Here's how the part is built. I have some questions about the finished solid (model axes, mm). Face numbers are marked on the shaded views. A direction names the side the tool comes from. Give positions to 0.01 mm unless a question says otherwise; leave off trailing zeros. Write each loop counter-clockwise with the first axis right and the second up, starting at its lowest first coordinate (ties: lowest second). Pieces come first, ordered by that corner, then holes. Notation, with made-up numbers: (52, 24) - (57, 24) arc R19 ccw to (57, 49) - close; hole circle Ø6 at (82, 69.5). An arc over 180 degrees is marked (long way). Use one line per item in the form item = value. Start each with the question number.
from build123d import *

# Parameters (mm, degrees)
BOSS_EXTRUDE1_DEPTH      = 4
BOSS_EXTRUDE1_DEPTH_BACK = 2


with BuildPart() as part:
    # Sketch3 → Boss-Extrude1 (new body, two sides)
    with BuildSketch(Plane.XY) as boss_extrude1_sk:
        with BuildLine():
            Line((-3.803846336, 5.696775672), (24.708284265, 24.734871916))
            ThreePointArc((24.708284265, 24.734871916), (65.032506622, 5.199104), (28.324251817, -20.49512037))
            Line((28.324251817, -20.49512037), (-2.850444576, -6.228761171))
            ThreePointArc((-2.850444576, -6.228761171), (-6.828213831, -0.545889982), (-3.803846336, 5.696775672))
        make_face()
        with BuildLine():
            Line((-3.526193319, 5.28095263), (24.985937282, 24.319048874))
            ThreePointArc((24.985937282, 24.319048874), (64.534096854, 5.159258016), (28.532313465, -20.04046627))
            Line((28.532313465, -20.04046627), (-2.642382928, -5.774107071))
            ThreePointArc((-2.642382928, -5.774107071), (-6.329804063, -0.506043998), (-3.526193319, 5.28095263))
        make_face(mode=Mode.SUBTRACT)
    extrude(amount=BOSS_EXTRUDE1_DEPTH)
    extrude(boss_extrude1_sk.sketch, amount=-BOSS_EXTRUDE1_DEPTH_BACK)


solid = part.part
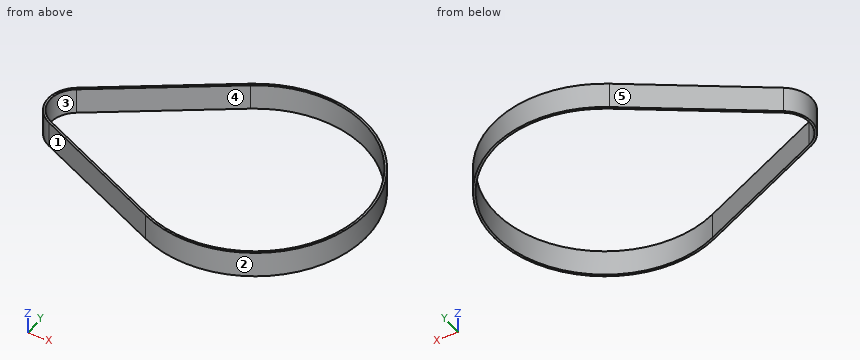
1. I want a section at C-C, the plane y = -3.5. List the corners of the cut face in (x, z) for me.
2. I want a section at A-A, the plane x = 59.5. List the corners of the cut face in (y, z) for me.
3. I want a section at B-B, the plane z = 2.9. List the corners of the cut face in (x, y) for me, then the cut area to 3 significant figures.
4. For P1, Ø1.5, axis at y = 21, z = 2.5, coming from the -X side; P2, Ø3, axis at y = -14.5, z = 0.5, coming from the +X side; P3, Ø1.5, axis at y = 7, z = 0.5, coming from the +X side, each with a flat end and sliding along its axis, tell me the tip position at first contact or that it passes through.
5. We'd pull the mould along X, two halves only. Please class the marked faces 1, 2 and 3: pulls with the +X half, pulls with the -X half, needs draft (parallel to the pull), parting line crosses it, or undercut.
6. For the marked faces 4 and 5, which set-ups out of +Z, -Z, +X, -X, +Y, -Y let a thin tool reach every point of the face, with its end or its side?
7. Please list where these lines run through material, in increasing order: line 1 (Y direction, x = 39, z = 0.1); line 2 (X direction, y = 0, z = 3.6); line 3 (X direction, y = 18, z = 0.1).
Result sheet:
q1.outline = (-5.89, -2) - (-5.3, -2) - (-5.3, 4) - (-5.89, 4) - close; (63.74, -2) - (64.26, -2) - (64.26, 4) - (63.74, 4) - close
q2.outline = (-13, -2) - (-12.18, -2) - (-12.18, 4) - (-13, 4) - close; (18.44, -2) - (19.26, -2) - (19.26, 4) - (18.44, 4) - close
q3.outline = (-3.8, 5.7) arc R6.85 ccw to (-2.85, -6.23) - (28.32, -20.5) arc R25.98 ccw (long way) to (24.71, 24.73) - close; hole (-3.53, 5.28) arc R6.35 ccw to (-2.64, -5.77) - (28.53, -20.04) arc R25.48 ccw (long way) to (24.99, 24.32) - close
q3.area = 94.8 mm2
q4.P1 = 17.99
q4.P2 = 59.5
q4.P3 = 64.93
q5.face_1 = pulls with the -X half
q5.face_2 = parting line crosses it
q5.face_3 = undercut
q6.face_4 = +Z, -Z
q6.face_5 = +Z, -Z, -X, +Y
q7.line_1 = -22.85 to -22.35, 28.61 to 29.11
q7.line_2 = -6.85 to -6.35, 64.42 to 64.93
q7.line_3 = 14.62 to 15.52, 59.83 to 60.44
